Can you work these out from the drawing? Everything is in mm from the part's minimum corner. A direction names the side the tool comes from. Coordinates: 2 decimals unless noted, no trailing zeros. Order: outer loops, then holes, each group sorted by start corner. A loop starts at its lowest first (then second) coordinate and runs counter-clockwise, first axis right, second up. Notation, with made-up numbers: (36.5, 48) -> (63.5, 48) arc R24 cw to (63.5, 83) -> close; hole circle Ø8 at (75, 25.25). An arc over 180 degrees is marked (long way). Put each result on its own line as item: value. Start each with the question number.
Q1. Will this pin go through, and if not, where does the flat tip stop? pin 1 (3 mm diameter, centred on y = 4.5, z = 10.5, fed in from +X).
Q2. For the marked faces 1, 2, 3, 4 and 5, which set-ups out of +Z, -Z, +X, -X, +Y, -Y let a thin tool reach every point of the face, with its end or its side?
Q3. If we section it at D-D (z = 11.25): Please give me the cut outline in (x, y).
Q4. Please list where these lines run through material, in increasing order: line 1 along X through (y, z) = (0.7, 2.5); line 2 along Y through (x, z) = (4.95, 3); line 3 along Z through (x, y) = (3.25, 4.9).
Q5. If we section it at A-A (z = 2.25): Please give me the cut outline in (x, y).
Q6. If we section it at C-C (y = 2.8): Please give me the cut outline in (x, z).
Q7. If we section it at B-B (x = 1.5): Please give me the cut outline in (y, z), and give its area (3 significant figures).
Q8. We'd pull the mould along Y, two halves only. Please class the marked faces 6, 7 and 8: +Y half, -Y half, draft (parallel to the pull), parting line (faces both ways), or undercut.
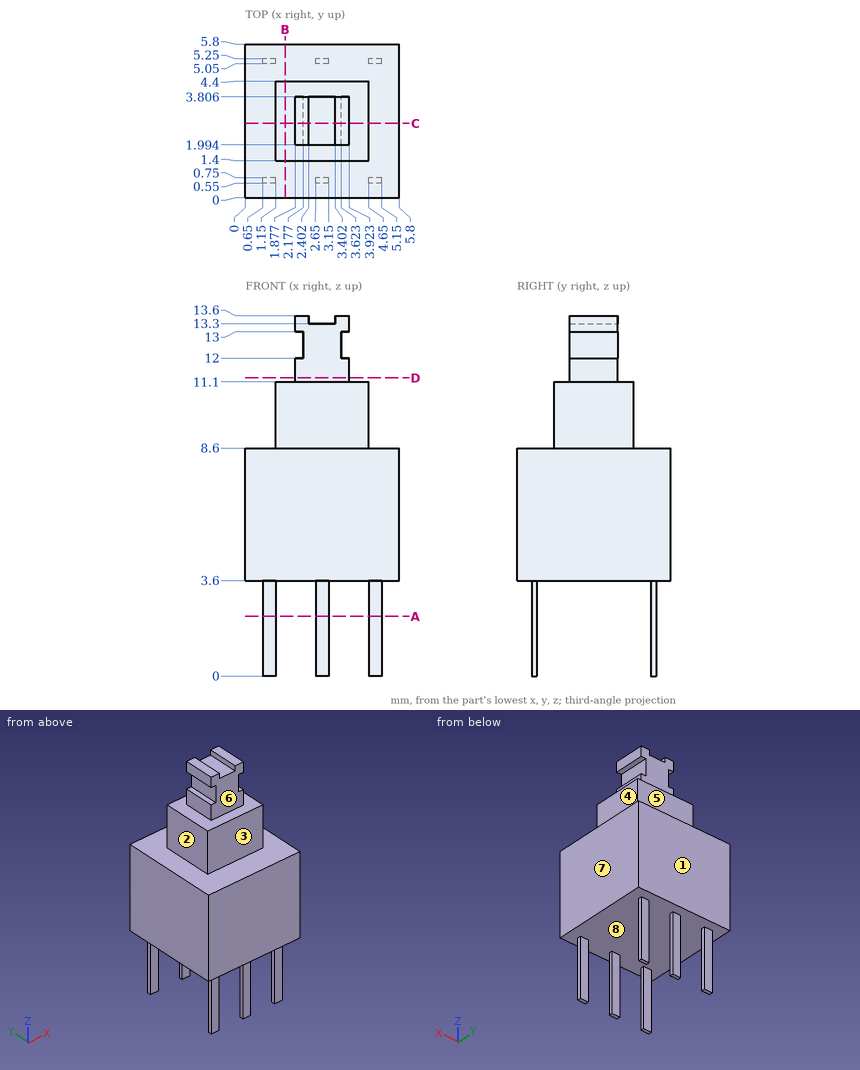
The answers:
1. pin 1: x = 4.65
2. face 1: +Z, -Z, +X, -X, +Y
2. face 2: +Z, -X, +Y, -Y
2. face 3: +Z, +X, -X, -Y
2. face 4: +Z, +X, +Y, -Y
2. face 5: +Z, +X, -X, +Y
3. outline: (1.88, 1.99) -> (3.92, 1.99) -> (3.92, 3.81) -> (1.88, 3.81) -> close
4. line 1: 0.65 to 1.15, 2.65 to 3.15, 4.65 to 5.15
4. line 2: 0.55 to 0.75, 5.05 to 5.25
4. line 3: 3.6 to 8.6
5. outline: (0.65, 0.55) -> (1.15, 0.55) -> (1.15, 0.75) -> (0.65, 0.75) -> close; (0.65, 5.05) -> (1.15, 5.05) -> (1.15, 5.25) -> (0.65, 5.25) -> close; (2.65, 0.55) -> (3.15, 0.55) -> (3.15, 0.75) -> (2.65, 0.75) -> close; (2.65, 5.05) -> (3.15, 5.05) -> (3.15, 5.25) -> (2.65, 5.25) -> close; (4.65, 0.55) -> (5.15, 0.55) -> (5.15, 0.75) -> (4.65, 0.75) -> close; (4.65, 5.05) -> (5.15, 5.05) -> (5.15, 5.25) -> (4.65, 5.25) -> close
6. outline: (0, 3.6) -> (5.8, 3.6) -> (5.8, 8.6) -> (4.65, 8.6) -> (4.65, 11.1) -> (3.92, 11.1) -> (3.92, 12) -> (3.62, 12) -> (3.62, 13) -> (3.92, 13) -> (3.92, 13.6) -> (3.4, 13.6) -> (3.4, 13.3) -> (2.4, 13.3) -> (2.4, 13.6) -> (1.88, 13.6) -> (1.88, 13) -> (2.18, 13) -> (2.18, 12) -> (1.88, 12) -> (1.88, 11.1) -> (1.15, 11.1) -> (1.15, 8.6) -> (0, 8.6) -> close
7. outline: (0, 3.6) -> (5.8, 3.6) -> (5.8, 8.6) -> (4.4, 8.6) -> (4.4, 11.1) -> (1.4, 11.1) -> (1.4, 8.6) -> (0, 8.6) -> close
7. area: 36.5 mm^2
8. face 6: -Y half
8. face 7: draft
8. face 8: undercut
